Read the model definition and answer for the solid it produces. Units are mm, in the model's axes. A direction names the side the tool comes from. Give positions to 0.01 mm unless a question says otherwise; leave off trailing zeros. Write each loop counter-clockwise with the first axis right and the second up, starting at its lowest first coordinate (ties: lowest second). Pieces come first, ordered by that corner, then holes. Notation, with made-up numbers: M 30.5,-19.75 L 76.5,-19.75 A5 ccw 76.5,-15.75 Z; hole C 25,32.25 d6. An arc over 180 degrees is marked long. Use a Markdown table: item, result. Add a question column.
Item 1: The mould has two halves that part along Z. Classify faces 1 (the flat face through (1087, -48, -85)), 2 (the flat face through (0, -1, -64)), 3 (the flat face through (1088, -45, -88)): pulls with the +Z half, pulls with the -Z half, needs draft (parallel to the pull), parting line crosses it, or undercut.
Item 2: A cutting plane is placed at C-C on z = -66.5. Determine the outline of the cut face in (x, y), then the cut area to 3 significant figures.
Item 3: A cutting plane is placed at A-A on x = 232.5. Determine the outline of the cut face in (y, z).
Item 4: For faces 4 (the flat face through (1088, -3, -42)), 5 (the flat face through (1090, 0, -42)), determine the directions among +Z, -Z, +X, -X, +Y, -Y from which every point of the face is accessible in a straight line to the end or side of a thin tool.
Item 5: Given P1, Ø1.5, axis at x = 1621, y = -9, coming from the +Z side, flat-ended and moving along its own axis, determine where the tip first touches the part or whether it passes through.
Item 6: Consider probe 1 along Z at (x, y) = (902, -82.5); probe 2 along Y at (x, z) = (1339.5, -26); probe 3 along Y at (x, z) = (1511.5, -83.5). Determine where each line is inside the solid, lowest interval first. Write a range as [from, to].
Item 7: A cutting plane is placed at B-B on y = -45.5. Determine the outline of the cut face in (x, z).
from build123d import *

# Parameters (mm, degrees)
BOSS_EXTRUDE1_DEPTH = 2210
FILLET1_R           = 3
CUT_EXTRUDE1_DEPTH  = 88


with BuildPart() as part:
    # Sketch1 → Boss-Extrude1 (new body)
    with BuildSketch(Plane(origin=(0, 0, 0), x_dir=(0, 0, -1), z_dir=(1, 0, 0))):
        Polygon((0, 0), (88, 0), (88, -88), (85, -88), (85, -3), (0, -3), align=None)
    extrude(amount=BOSS_EXTRUDE1_DEPTH)

    # Fillet1
    fillet1_edges = [part.edges().sort_by_distance(p)[0] for p in [
        (1105, 0, -88),
        (1105, -3, -85),
    ]]
    fillet(fillet1_edges, radius=FILLET1_R)

    # Sketch2 → Cut-Extrude1 (cut)
    with BuildSketch(Plane(origin=(0, 0, -88), x_dir=(-1, 0, 0), z_dir=(0, 0, -1))):
        Polygon((-2210, 0), (-2122, -88), (-2210, -88), align=None)
    extrude(amount=-CUT_EXTRUDE1_DEPTH, mode=Mode.SUBTRACT)


solid = part.part
Filled in:
| question | item | result |
|---|---|---|
| 1 | face 1 | pulls with the +Z half |
| 1 | face 2 | needs draft |
| 1 | face 3 | pulls with the -Z half |
| 2 | outline | M 0,-3 L 2207,-3 L 2210,0 L 0,0 Z |
| 2 | area | 6,630 mm² |
| 3 | outline | M -88,-88 L -3,-88 A3 ccw 0,-85 L 0,0 L -3,0 L -3,-82 A3 cw -6,-85 L -88,-85 Z |
| 4 | face 4 | +Z, +X, -X, -Y |
| 4 | face 5 | +Z, -Z, +X, -X, +Y |
| 5 | P1 | z = -85 |
| 6 | probe 1 | [-88, -85] |
| 6 | probe 2 | [-3, 0] |
| 6 | probe 3 | [-3.4, 0] |
| 7 | outline | M 0,-88 L 2164.5,-88 L 2164.5,-85 L 0,-85 Z |
